Geometry check sheet. Reference: the model listing, model coordinates, mm. A direction names the side the tool comes from. Give positions to 0.01 mm unless a question says otherwise; leave off trailing zeros. Order: outer loops, then holes, each group sorted by start corner. A loop starts at its lowest first (then second) coordinate and runs counter-clockwise, first axis right, second up. Notation, with made-up numbers: (23, 67.5) - (45, 67.5) arc R9 ccw to (45, 83.5) - close; hole circle Ø2 at (13.5, -39). An arc over 180 degrees is marked (long way). Put each result on its own line as item: value. Start each with the question number.
```python
from build123d import *

# Parameters (mm, degrees)
SKETCH1_W           = 59
SKETCH1_H           = 49.5
SKETCH1_R           = 3
BOSS_EXTRUDE1_DEPTH = 1.5
BOSS_EXTRUDE2_DEPTH = 49.5
CUT_EXTRUDE1_DEPTH  = 1
CUT_EXTRUDE3_DEPTH  = 65.105869466
BOSS_EXTRUDE3_START = 0.5
SKETCH5_R           = 3
BOSS_EXTRUDE3_DEPTH = 0.5
SKETCH6_W           = 3.5
SKETCH6_H           = 2.563301414
CUT_EXTRUDE4_DEPTH  = 0.5
CHAMFER3_SIZE       = 1.5
SKETCH7_W           = 59
SKETCH7_H           = 2.086537977
CUT_EXTRUDE5_DEPTH  = 58.762444547


with BuildPart() as part:
    # Sketch1 → Boss-Extrude1 (new body)
    with BuildSketch(Plane(origin=(0, 0, 0), x_dir=(1, 0, 0), z_dir=(0, 1, 0))):
        Rectangle(SKETCH1_W, SKETCH1_H)
        with Locations(Location((0, 0, 0), (0, 0, 270))):
            Circle(SKETCH1_R, mode=Mode.SUBTRACT)
    extrude(amount=BOSS_EXTRUDE1_DEPTH)

    # Sketch2 → Boss-Extrude2 (add)
    with BuildSketch(Plane(origin=(0, 0, -24.75), x_dir=(-1, 0, 0), z_dir=(0, 0, -1))):
        Polygon((-29.5, 1.5), (29.5, 1.5), (29.5, 2.5), (28.32, 4), (27.14, 2.5), (25.96, 4), (24.78, 2.5), (23.6, 4), (22.42, 2.5), (21.24, 4), (20.06, 2.5), (18.88, 4), (17.7, 2.5), (16.52, 4), (15.34, 2.5), (14.16, 4), (12.98, 2.5), (11.8, 4), (10.62, 2.5), (9.44, 4), (8.26, 2.5), (7.08, 4), (5.9, 2.5), (4.72, 4), (3.54, 2.5), (2.36, 4), (1.18, 2.5), (0, 4), (-1.18, 2.5), (-2.36, 4), (-3.54, 2.5), (-4.72, 4), (-5.9, 2.5), (-7.08, 4), (-8.26, 2.5), (-9.44, 4), (-10.62, 2.5), (-11.8, 4), (-12.98, 2.5), (-14.16, 4), (-15.34, 2.5), (-16.52, 4), (-17.7, 2.5), (-18.88, 4), (-20.06, 2.5), (-21.24, 4), (-22.42, 2.5), (-23.6, 4), (-24.78, 2.5), (-25.96, 4), (-27.14, 2.5), (-28.32, 4), (-29.5, 2.5), align=None)
    extrude(amount=-BOSS_EXTRUDE2_DEPTH)

    # Sketch3 → Cut-Extrude1 (cut)
    with BuildSketch(Plane(origin=(0, 0, 0), x_dir=(-1, 0, 0), z_dir=(0, -1, 0))):
        with BuildLine():
            Line((-1.75, -2.436698586), (-1.75, -5))
            Line((-1.75, -5), (1.75, -5))
            Line((1.75, -5), (1.75, -2.436698586))
            ThreePointArc((1.75, -2.436698586), (0, 3), (-1.75, -2.436698586))
        make_face()
    extrude(amount=-CUT_EXTRUDE1_DEPTH, mode=Mode.SUBTRACT)

    # Sketch4 → Cut-Extrude3 (cut, through all)
    with BuildSketch(Plane(origin=(29.5, 0, 0), x_dir=(0, 0, -1), z_dir=(1, 0, 0))):
        with BuildLine():
            Line((-24, 4), (-24.75, 4))
            Line((-24.75, 4), (-24.75, 3.25))
            ThreePointArc((-24.75, 3.25), (-24.530330086, 3.780330086), (-24, 4))
        make_face()
    cut_extrude3 = extrude(amount=-CUT_EXTRUDE3_DEPTH, mode=Mode.SUBTRACT)

    # Mirror1: Cut-Extrude3 across plane
    add(cut_extrude3.mirror(Plane.XY), mode=Mode.SUBTRACT)

    # Sketch5 → Boss-Extrude3 (add)
    with BuildSketch(Plane.XZ.offset(-1.5).offset(BOSS_EXTRUDE3_START)):
        Circle(SKETCH5_R)
    extrude(amount=-BOSS_EXTRUDE3_DEPTH)

    # Sketch6 → Cut-Extrude4 (cut)
    with BuildSketch(Plane.XZ.offset(-1)):
        with Locations((0, 3.718349293)):
            Rectangle(SKETCH6_W, SKETCH6_H)
    extrude(amount=-CUT_EXTRUDE4_DEPTH, mode=Mode.SUBTRACT)

    # Chamfer3
    chamfer3_edges = [part.edges().sort_by_distance(p)[0] for p in [
        (0, 0, 5),
    ]]
    chamfer(chamfer3_edges, length=CHAMFER3_SIZE - 0.0001)  # a hair under: the kernel refuses the full size

    # Sketch7 → Cut-Extrude5 (cut, through all)
    with BuildSketch(Plane.XY.offset(24.75)):
        with Locations((0, 3.543268988)):
            Rectangle(SKETCH7_W, SKETCH7_H)
    extrude(amount=-CUT_EXTRUDE5_DEPTH, mode=Mode.SUBTRACT)


solid = part.part
```
Item 1: Set-up check for faces 4 (the face through (-29.5, 1, 0)), 5 (the face through (-1.75, 1, 4)): record each of +Z, -Z, +X, -X, +Y, -Y from which the full face is reachable in a straight line by a thin tool's end or side.
Item 2: Cross-section at A-A (z = 0). Enter the section's corners in (x, y).
Item 3: Release check for a two-part mould opening along Z. For faces 1 (the face through (0, 0.7, 5.8)), 2 (the face through (0, 1, -24.75)), 3 (the face through (29.5, 1, 0)) record: +Z half, -Z half, draft (parallel to the pull), parting line (faces both ways), or undercut.
Item 4: Thickness scan on line 1 along X through (y, z) = (0.6, 0); line 2 along X through (y, z) = (1.15, 3.5); line 3 along Y through (x, z) = (-1.5, 2). Record the ranges inside material, lowest first.
Recorded:
1. face 4: +Z, -Z, -X, +Y, -Y
1. face 5: -Y
2. outline: (-29.5, 0) - (-3, 0) - (-3, 1) - (3, 1) - (3, 0) - (29.5, 0) - (29.5, 2.5) - (-29.5, 2.5) - close
3. face 1: undercut
3. face 2: -Z half
3. face 3: draft
4. line 1: x = -29.5 to -3, 3 to 29.5
4. line 2: x = -29.5 to -1.75, 1.75 to 29.5
4. line 3: y = 1 to 2.5
